Geometry check sheet. Reference: the model listing, model coordinates, mm. A direction names the side the tool comes from. Coordinates: 2 decimals unless noted, no trailing zeros. Order: outer loops, then holes, each group sorted by start corner. A loop starts at its lowest first (then second) coordinate and runs counter-clockwise, first axis right, second up. Notation, with made-up numbers: (2, -4) - (22, -4) arc R35 cw to (22, 28) - close; hole circle Ø8 at (59, 48). An arc over 180 degrees is marked (long way). Return JSON: item names as keys, results as strings. Group by question number.
Item 1: Gauge pin test, flat ends, axial feed: pin 1 (7 mm diameter, centred on y = -42, z = 16, fed in from +X); pin 2 (3.5 mm diameter, centred on y = -5.5, z = 18, fed in from -X); pin 3 (12.5 mm diameter, centred on x = -59, y = -23.5, fed in from +Z); pin 4 (10 mm diameter, centred on x = -50.8, z = -4.88, fed in from +Y). Record the tip position at first contact, or that the pin passes through.
Item 2: Tool access check on faces 1 (the flat face through (-55, 0, 2)), 2 (the flat face through (-25.4, -25, 5)), 3 (the flat face through (-63.5, -44, 17)), 4 (the flat face through (-82, -25, -4.722)). Record the directions out of +Z, -Z, +X, -X, +Y, -Y that give a thin tool (end or side, any length) a straight path to the whole face; none if there is none.
Item 3: Scan lines: probe 1 along Z at (x, y) = (-50.8, -16.5); probe 2 along Y at (x, z) = (-67.5, 15); probe 3 along Z at (x, y) = (-50.8, -38.5). Record each from-to range of solid material in increasing order.
Item 4: Section check A-A on z = 11. Enter the section's corners in (x, y), then the cut area to 3 significant figures.
Item 5: Section check B-B on x = -50.8. Enter the section's corners in (y, z).
Item 6: Section check D-D on x = -27. Enter the section's corners in (y, z), then the cut area to 3 significant figures.
Item 7: Section check C-C on y = -15.5. Enter the section's corners in (x, z).
Item 8: Draft check along Z on faces 5 (the flat face through (-50, -38.1, 13)), 6 (the cylindrical face through (-44.934, -25.044, -7.317)), 7 (the flat face through (-32, -44, 20.678)). Enter one of: pulls with the +Z half, pulls with the -Z half, needs draft (parallel to the pull), parting line crosses it, or undercut.
from build123d import *

# Parameters (mm, degrees)
F1_DEPTH = 50.8
F2_R     = 6.35
F3_DEPTH = 50.801
F4_W     = 25.4
F4_H     = 12.7
F5_DEPTH = 88.901


with BuildPart() as f1:
    # F0 (on Front) → F1 (new body)
    with BuildSketch(Plane.XZ):
        Polygon((-76.2, -4.721795), (-88.9, -4.721795), (-88.9, -17.421795), (0, -17.421795), (0, -4.721795), (-25.4, -4.721795), (-25.4, 20.678205), (-38.1, 20.678205), (-38.1, 14.165386), (-63.5, 14.165386), (-63.5, 20.678205), (-76.2, 20.678205), align=None)
    extrude(amount=F1_DEPTH)

    # F2 (on Front) → F3 (cut, through all)
    with BuildSketch(Plane.XZ):
        with Locations((-50.8, -4.884614)):
            Circle(F2_R)
    extrude(amount=F3_DEPTH, mode=Mode.SUBTRACT)

    # F4 (on Right) → F5 (cut, through all)
    with BuildSketch(Plane.YZ):
        with Locations((-25.4, 14.328205)):
            Rectangle(F4_W, F4_H)
    extrude(amount=-F5_DEPTH, mode=Mode.SUBTRACT)


solid = f1.part
Computed:
{
 "1": {"pin 1": "stops at x = -25.4", "pin 2": "stops at x = -76.2", "pin 3": "stops at z = 7.98", "pin 4": "passes through"},
 "2": {"face 1": "+Z, -Z, +X, -X, +Y", "face 2": "+Z, +X, +Y, -Y", "face 3": "+Z, +Y, -Y", "face 4": "+Z, -X, +Y, -Y"},
 "3": {"probe 1": "z = -17.42 to -11.23, 1.47 to 7.98", "probe 2": "y = -50.8 to -38.1, -12.7 to 0", "probe 3": "z = -17.42 to -11.23, 1.47 to 14.17"},
 "4": {"outline": "(-76.2, -50.8) - (-25.4, -50.8) - (-25.4, -38.1) - (-76.2, -38.1) - close; (-76.2, -12.7) - (-25.4, -12.7) - (-25.4, 0) - (-76.2, 0) - close", "area": "1,290 mm²"},
 "5": {"outline": "(-50.8, -17.42) - (0, -17.42) - (0, -11.23) - (-50.8, -11.23) - close; (-50.8, 1.47) - (0, 1.47) - (0, 14.17) - (-12.7, 14.17) - (-12.7, 7.98) - (-38.1, 7.98) - (-38.1, 14.17) - (-50.8, 14.17) - close"},
 "6": {"outline": "(-50.8, -17.42) - (0, -17.42) - (0, 20.68) - (-12.7, 20.68) - (-12.7, 7.98) - (-38.1, 7.98) - (-38.1, 20.68) - (-50.8, 20.68) - close", "area": "1,610 mm²"},
 "7": {"outline": "(-88.9, -17.42) - (0, -17.42) - (0, -4.72) - (-25.4, -4.72) - (-25.4, 7.98) - (-76.2, 7.98) - (-76.2, -4.72) - (-88.9, -4.72) - close; hole circle Ø12.7 at (-50.8, -4.88)"},
 "8": {"face 5": "needs draft", "face 6": "undercut", "face 7": "pulls with the +Z half"}
}
